The listing builds one solid part. Answer for the finished solid, in the listing's coordinates (mm). Round coordinates to 2 decimals unless told otherwise and drop trailing zeros. Loops run counter-clockwise (first coordinate to the right, second up) from the corner with the lowest first, then second, coordinate; pieces in that order, holes last. Notation, with made-up numbers: (51.25, 68) - (79.25, 68) arc R22 cw to (79.25, 84) - close; hole circle Ø11 at (39.5, -7.5). An arc over 180 degrees is marked (long way). Write item = value, one per line. Start each with the question number.
1) Given pin 1 Ø1 at (x, z) = (87, 1) entering from -Y; pin 2 Ø3 at (x, y) = (115.18, 66.5) entering from +Z; pin 3 Ø1 at (y, z) = (-100.5, 1) entering from -X, each flat-ended and moving along its own axis, determine where each tip first touches the part or whether it passes through.
2) Section B-B, the plane x = -124 is taken. Determine the outline of the cut face in (y, z), and give its area (3 significant figures).
3) Section C-C, the plane y = -56.5 is taken. Determine the outline of the cut face in (x, z).
4) Section A-A, the plane z = 1.85 is taken. Determine the outline of the cut face in (x, y), and give its area (3 significant figures).
5) Straight lines are drawn through the part: line 1 along Y through (x, z) = (0, 0.75); line 2 along X through (y, z) = (-133, 1.9); line 3 along X through (y, z) = (66.5, 1.1). For each, find the intervals that lie inside material, in ascending order.
from build123d import *

# Parameters (mm, degrees)
SALIENTE_EXTRUIR1_DEPTH = 3
REDONDEO1_R             = 20
CROQUIS2_R              = 1.75
CORTAR_EXTRUIR1_DEPTH   = 212.545651301


with BuildPart() as part:
    # Croquis1 → Saliente-Extruir1 (new body)
    with BuildSketch(Plane.XY):
        Polygon((-80.829037687, -140), (80.829037687, -140), (161.658075373, 0), (80.829037687, 140), (-80.829037687, 140), (-161.658075373, 0), align=None)
    extrude(amount=SALIENTE_EXTRUIR1_DEPTH)

    # Redondeo1
    redondeo1_edges = [part.edges().sort_by_distance(p)[0] for p in [
        (161.658075373, 0, 1.5),
        (80.829037687, -140, 1.5),
        (-80.829037687, -140, 1.5),
        (-161.658075373, 0, 1.5),
        (-80.829037687, 140, 1.5),
        (80.829037687, 140, 1.5),
    ]]
    fillet(redondeo1_edges, radius=REDONDEO1_R)

    # Croquis2 → Cortar-Extruir1 (cut, through all)
    with BuildSketch(Plane(origin=(0, 0, 0), x_dir=(1, 0, 0), z_dir=(0, 0, -1))):
        with Locations(Location((0, 133, 0), (0, 0, 180))):
            Circle(CROQUIS2_R)
        with Locations(Location((115.181378703, -66.5, 0), (0, 0, 180))):
            Circle(CROQUIS2_R)
        with Locations(Location((-115.181378703, -66.5, 0), (0, 0, 180))):
            Circle(CROQUIS2_R)
    extrude(amount=-CORTAR_EXTRUIR1_DEPTH, mode=Mode.SUBTRACT)


solid = part.part
Geometry check:
q1.pin_1 = -130.18
q1.pin_2 = through
q1.pin_3 = -103.92
q2.outline = (-65.23, 0) - (65.23, 0) - (65.23, 3) - (-65.23, 3) - close
q2.area = 391 mm2
q3.outline = (-129.04, 0) - (129.04, 0) - (129.04, 3) - (-129.04, 3) - close
q4.outline = (-155.88, -10) - (-86.6, -130) arc R20 ccw to (-69.28, -140) - (69.28, -140) arc R20 ccw to (86.6, -130) - (155.88, -10) arc R20 ccw to (155.88, 10) - (86.6, 130) arc R20 ccw to (69.28, 140) - (-69.28, 140) arc R20 ccw to (-86.6, 130) - (-155.88, 10) arc R20 ccw to start; hole circle Ø3.5 at (-115.18, 66.5); hole circle Ø3.5 at (0, -133); hole circle Ø3.5 at (115.18, 66.5)
q4.area = 67,700 mm2
q5.line_1 = -140 to -134.75, -131.25 to 140
q5.line_2 = -84.48 to -1.75, 1.75 to 84.48
q5.line_3 = -123.26 to -116.93, -113.43 to 113.43, 116.93 to 123.26
